Study the drawing (mm; zero at the part's minimum x, y, z) and answer. A direction names the side the tool comes from. Coordinates: 2 decimals unless noted, no trailing zeros. Order: outer loops, then holes, each group sorted by start corner. A loop starts at its lowest first (then second) coordinate and runs counter-clockwise, first axis right, second up.
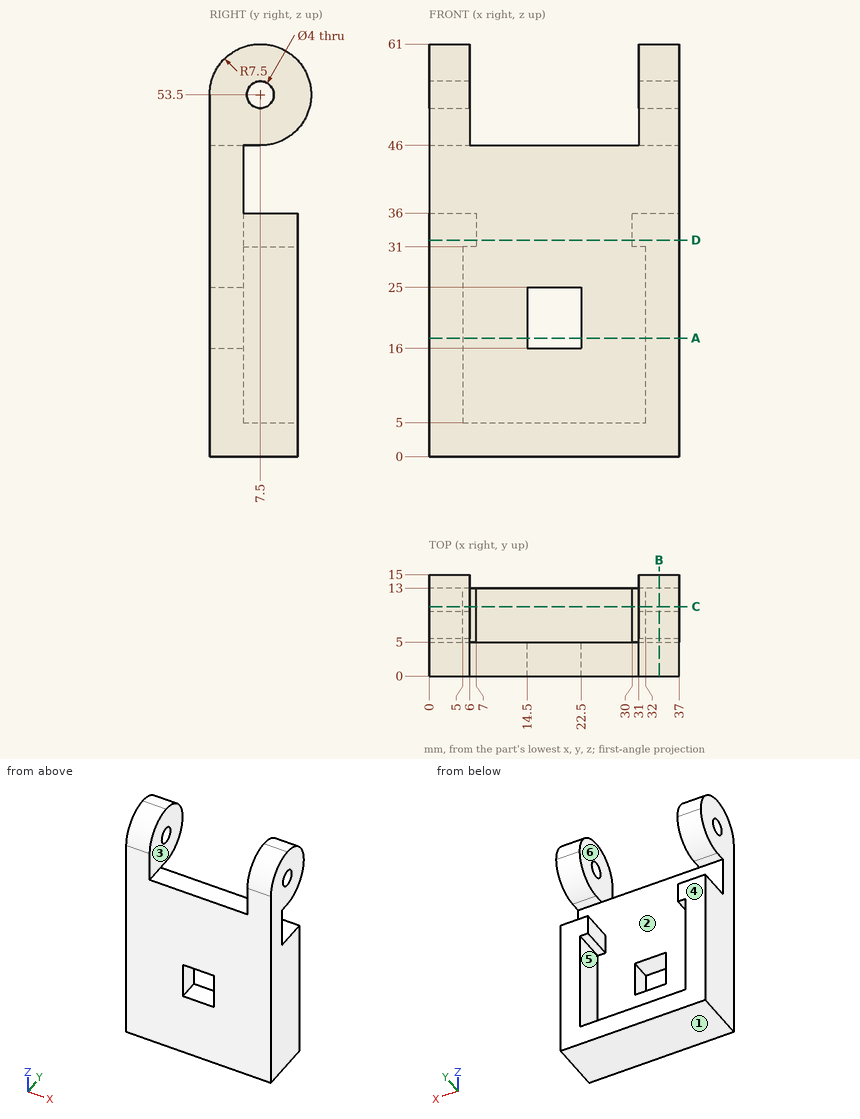
1) A cutting plane is placed at B-B, the plane x = 34. Determine the outline of the cut face in (y, z).
A:
outline: (0, 0) - (13, 0) - (13, 36) - (5, 36) - (5, 46) - (7.5, 46) arc R7.5 ccw (long way) to (0, 53.5) - close; hole circle Ø4 at (7.5, 53.5)
2) Determine the mould class of the marked faces 1, 2 and 3 for opening direction Z: pulls with the +Z half, pulls with the -Z half, needs draft (parallel to the pull), parting line crosses it, or undercut.
A:
face 1: pulls with the -Z half
face 2: undercut
face 3: needs draft
3) A cutting plane is placed at D-D, the plane z = 32. Determine the outline of the cut face in (x, y), and give its area (3 significant figures).
A:
outline: (0, 0) - (37, 0) - (37, 13) - (30, 13) - (30, 5) - (7, 5) - (7, 13) - (0, 13) - close
area: 297 mm2
4) Which of the six approach directions +Z, -Z, +X, -X, +Y, -Y give full straight-line access (tool end or side, diameter ignored) to the marked faces 4, 5 and 6?
A:
face 4: -Z, +X, -X, +Y
face 5: +Y
face 6: +Z, +Y, -Y
5) A cutting plane is placed at C-C, the plane y = 10.25. Determine the outline of the cut face in (x, z), and give its area (3 significant figures).
A:
outline: (0, 0) - (37, 0) - (37, 36) - (30, 36) - (30, 31) - (32, 31) - (32, 5) - (5, 5) - (5, 31) - (7, 31) - (7, 36) - (0, 36) - close; (0, 46.52) - (6, 46.52) - (6, 60.48) - (0, 60.48) - close; (31, 46.52) - (37, 46.52) - (37, 60.48) - (31, 60.48) - close
area: 682 mm2
6) A cutting plane is placed at A-A, the plane z = 17.5. Determine the outline of the cut face in (x, y).
A:
outline: (0, 0) - (14.5, 0) - (14.5, 5) - (5, 5) - (5, 13) - (0, 13) - close; (22.5, 0) - (37, 0) - (37, 13) - (32, 13) - (32, 5) - (22.5, 5) - close
7) Straight lines are drawn through the part: line 1 (Y direction, x = 2.05, z = 53.5); line 2 (X direction, y = 4.5, z = 55); line 3 (Z direction, x = 28, y = 10). For each, find the intervals that lie inside material, in ascending order.
A:
line 1: y = 0 to 5.5, 9.5 to 15
line 2: x = 0 to 6, 31 to 37
line 3: z = 0 to 5
8) Flat-ended cylindrical pins translate along their axes: pin 1 Ø4 at (x, y) = (20, 3.5) entering from +Z; pin 2 Ø4 at (x, y) = (16, 10) entering from +Z; pin 3 Ø1 at (x, z) = (9, 12.5) entering from +Y. Find the tip coordinate at first contact, or state that the pin passes through.
A:
pin 1: stops at z = 46
pin 2: stops at z = 5
pin 3: stops at y = 5
